Geometry check sheet. Reference: the model listing, model coordinates, mm. A direction names the side the tool comes from. Round coordinates to 2 decimals unless told otherwise and drop trailing zeros. Write each loop counter-clockwise with the first axis right and the second up, starting at its lowest first coordinate (ties: lowest second). Pieces come first, ordered by that corner, then holes. Notation, with made-up numbers: (-15.75, -29) - (5.25, -29) arc R25 cw to (5.25, 2) - close; hole circle Ø5 at (4, 24.25). An arc over 180 degrees is marked (long way). Return JSON: item names as keys, results as strings.
```python
from build123d import *

# Parameters (mm, degrees)
CUT_EXTRUDE_1_DEPTH = 30


with BuildPart() as part:
    # 草图1 → 旋转2 (revolve)
    with BuildSketch(Plane.XY, mode=Mode.PRIVATE) as revolve_2_sk:
        Polygon((0, 2), (0, 0), (17, 0), (21, 0), (21, 2), (17, 2), (17, 4), (4, 4), (4, 2), align=None)
    revolve(revolve_2_sk.sketch.rotate(Axis((-16.701754386, 0, 0), (1, 0, 0)), 180), axis=Axis((-16.701754386, 0, 0), (1, 0, 0)))

    # 草图2 → 切除-拉伸1 (cut)
    with BuildSketch(Plane(origin=(0, 0, 0), x_dir=(1, 0, 0), z_dir=(0, 1, 0))):
        with BuildLine():
            ThreePointArc((11.5, 0), (10.5, 1), (9.5, 0))
            Line((9.5, 0), (11.5, 0))
        make_face()
        with BuildLine():
            Line((11.5, 0), (9.5, 0))
            ThreePointArc((9.5, 0), (10.5, -1), (11.5, 0))
        make_face()
    extrude(amount=-CUT_EXTRUDE_1_DEPTH, mode=Mode.SUBTRACT)


solid = part.part
```
(1) Section check B-B, the plane z = 0. Enter the section's corners in (x, y).
Response values:
{"outline": "(0, -2) - (4, -2) - (4, -4) - (9.5, -4) - (9.5, 0) - (11.5, 0) - (11.5, -4) - (17, -4) - (17, -2) - (21, -2) - (21, 2) - (17, 2) - (17, 4) - (4, 4) - (4, 2) - (0, 2) - close"}
(2) Section check D-D, the plane z = 1.5. Enter the section's corners in (x, y), plus the area to 3 significant figures.
Response values:
{"outline": "(0, -1.32) - (4, -1.32) - (4, -3.71) - (17, -3.71) - (17, -1.32) - (21, -1.32) - (21, 1.32) - (17, 1.32) - (17, 3.71) - (4, 3.71) - (4, 1.32) - (0, 1.32) - close", "area": "118 mm^2"}
(3) Material ranges on line 1 along X through (y, z) = (2, 1.5); line 2 along Z through (x, y) = (10.5, -2.95); line 3 along Z through (x, y) = (10.5, -3.2), recorded low to high. Write a range as [from, to].
Response values:
{"line 1": "x = [4, 17]", "line 2": "z = [-2.7, -1], [1, 2.7]", "line 3": "z = [-2.4, -1], [1, 2.4]"}
(4) Gauge pin test, flat ends, axial feed: pin 1 (1.8 mm diameter, centred on x = 10.5, z = 0, fed in from -Y); pin 2 (4 mm diameter, centred on x = 2.5, y = 1.5, fed in from +Z); pin 3 (2 mm diameter, centred on y = 1.5, z = -3, fed in from +X). Record the tip position at first contact, or that the pin passes through.
Response values:
{"pin 1": "stops at y = 0", "pin 2": "stops at z = 4", "pin 3": "stops at x = 17"}
(5) Release check for a two-part mould opening along Z. For faces 1 (the face through (4, 2, 1)), 2 (the face through (10, 0, 0)), 3 (the face through (11.3, -2, -0.6)), 4 (the face through (10.409, 0.867, 3.905)) record: pulls with the +Z half, pulls with the -Z half, needs draft (parallel to the pull), parting line crosses it, or undercut.
Response values:
{"face 1": "needs draft", "face 2": "undercut", "face 3": "undercut", "face 4": "parting line crosses it"}
(6) Section check C-C, the plane x = 16.75. Enter the section's corners in (y, z).
Response values:
{"outline": "circle Ø8 at (0, 0)"}
(7) Section check A-A, the plane y = -0.75. Enter the section's corners in (x, z), plus the area to 3 significant figures.
Response values:
{"outline": "(0, -1.85) - (4, -1.85) - (4, -3.93) - (17, -3.93) - (17, -1.85) - (21, -1.85) - (21, 1.85) - (17, 1.85) - (17, 3.93) - (4, 3.93) - (4, 1.85) - (0, 1.85) - close; hole circle Ø2 at (10.5, 0)", "area": "129 mm^2"}
(8) Access from +Z, -Z, +X, -X, +Y, -Y to the whole of each face (thin tool, end or side, straight path). Record for faces 5 (the face through (21, 0, 0)), 6 (the face through (2, 0, 2)), 7 (the face through (17, 1, -2)).
Response values:
{"face 5": "+Z, -Z, +X, +Y, -Y", "face 6": "-X", "face 7": "+X"}
